```python
from build123d import *

# Parameters (mm, degrees)
SKETCH1_R           = 51.5
BOSS_EXTRUDE1_DEPTH = 2
SKETCH2_R           = 17.25
CUT_EXTRUDE1_DEPTH  = 2
BOSS_EXTRUDE3_START = 6
BOSS_EXTRUDE3_DEPTH = 6
CIRPATTERN2_COUNT   = 6
BOSS_EXTRUDE4_START = 6
SKETCH5_R           = 19.5
SKETCH5_R_2         = 17.25
BOSS_EXTRUDE4_DEPTH = 6
CHAMFER1_SIZE       = 1
CHAMFER1_SIZE2      = 3
BOSS_EXTRUDE5_START = 2
SKETCH6_R           = 51.5
BOSS_EXTRUDE5_DEPTH = 2
SKETCH7_R           = 19.5
BOSS_EXTRUDE6_DEPTH = 5
SKETCH8_R           = 9.5
BOSS_EXTRUDE7_DEPTH = 28
CUT_EXTRUDE2_DEPTH  = 79.028840822
SKETCH10_R          = 7.5
CUT_EXTRUDE3_DEPTH  = 2
SKETCH11_R          = 15.5
SKETCH11_R_2        = 12.5
CUT_EXTRUDE4_DEPTH  = 3
SKETCH12_R          = 57.826662367
SKETCH12_R_2        = 50.5
CUT_EXTRUDE5_DEPTH  = 50


with BuildPart() as part:
    # Sketch1 → Boss-Extrude1 (new body)
    with BuildSketch(Plane.XY):
        Circle(SKETCH1_R)
    extrude(amount=BOSS_EXTRUDE1_DEPTH)

    # Sketch2 → Cut-Extrude1 (cut)
    with BuildSketch(Plane.XY.offset(2)):
        Circle(SKETCH2_R)
    extrude(amount=-CUT_EXTRUDE1_DEPTH, mode=Mode.SUBTRACT)

    # Sketch4 → Boss-Extrude3 (add)
    with BuildSketch(Plane(origin=(0, 0, 0), x_dir=(-1, 0, 0), z_dir=(0, 0, -1)).offset(BOSS_EXTRUDE3_START)):
        with BuildLine():
            Line((15.659504395, 12.715698759), (12.020980416, 14.553474713))
            ThreePointArc((12.020980416, 14.553474713), (-0.569243838, 34.9508437), (-21.374545455, 46.854869615))
            ThreePointArc((-21.374545455, 46.854869615), (-19.207405538, 47.784156082), (-17, 48.613269793))
            ThreePointArc((-17, 48.613269793), (3.810982012, 34.741493963), (15.659504395, 12.715698759))
        make_face()
    boss_extrude3 = extrude(amount=-BOSS_EXTRUDE3_DEPTH)

    # CirPattern2: Boss-Extrude3 ×6 about axis
    cirpattern2_axis = Axis((0, 0, 0), (0, 0, 1))
    for i in range(1, CIRPATTERN2_COUNT):
        add(boss_extrude3.rotate(cirpattern2_axis, i * 360 / CIRPATTERN2_COUNT))

    # Sketch5 → Boss-Extrude4 (add)
    with BuildSketch(Plane.XY.offset(2).offset(BOSS_EXTRUDE4_START)):
        Circle(SKETCH5_R)
        Circle(SKETCH5_R_2, mode=Mode.SUBTRACT)
    extrude(amount=-BOSS_EXTRUDE4_DEPTH)

    # Chamfer1
    chamfer1_edges = [part.edges().sort_by_distance(p)[0] for p in [
        (-17.25, 0, 8),
    ]]
    chamfer1_side = [part.faces().sort_by_distance(p)[0] for p in [
        (-18.948456711, 0, 8),
    ]]
    chamfer(chamfer1_edges, length=CHAMFER1_SIZE, length2=CHAMFER1_SIZE2, reference=chamfer1_side[0])

    # Sketch6 → Boss-Extrude5 (add)
    with BuildSketch(Plane(origin=(0, 0, -6), x_dir=(-1, 0, 0), z_dir=(0, 0, -1)).offset(BOSS_EXTRUDE5_START)):
        Circle(SKETCH6_R)
    extrude(amount=-BOSS_EXTRUDE5_DEPTH)

    # Sketch7 → Boss-Extrude6 (add)
    with BuildSketch(Plane(origin=(0, 0, -8), x_dir=(-1, 0, 0), z_dir=(0, 0, -1))):
        with Locations(Location((0, 0, 0), (0, 0, 180))):
            Circle(SKETCH7_R)
    extrude(amount=BOSS_EXTRUDE6_DEPTH)

    # Sketch8 → Boss-Extrude7 (add)
    with BuildSketch(Plane(origin=(0, 0, -13), x_dir=(-1, 0, 0), z_dir=(0, 0, -1))):
        Circle(SKETCH8_R)
    extrude(amount=-BOSS_EXTRUDE7_DEPTH)

    # Sketch9 → Cut-Extrude2 (cut, through all)
    with BuildSketch(Plane.XY.offset(15)):
        with BuildLine():
            Line((6, 0), (6, 3.605551275))
            ThreePointArc((6, 3.605551275), (0, 7), (-6, 3.605551275))
            Line((-6, 3.605551275), (-6, 0))
            Line((-6, 0), (-6, -3.605551275))
            ThreePointArc((-6, -3.605551275), (0, -7), (6, -3.605551275))
            Line((6, -3.605551275), (6, 0))
        make_face()
    extrude(amount=-CUT_EXTRUDE2_DEPTH, mode=Mode.SUBTRACT)

    # Sketch10 → Cut-Extrude3 (cut)
    with BuildSketch(Plane(origin=(0, 0, -13), x_dir=(-1, 0, 0), z_dir=(0, 0, -1))):
        Circle(SKETCH10_R)
    extrude(amount=-CUT_EXTRUDE3_DEPTH, mode=Mode.SUBTRACT)

    # Sketch11 → Cut-Extrude4 (cut)
    with BuildSketch(Plane(origin=(0, 0, -13), x_dir=(-1, 0, 0), z_dir=(0, 0, -1))):
        Circle(SKETCH11_R)
        Circle(SKETCH11_R_2, mode=Mode.SUBTRACT)
    extrude(amount=-CUT_EXTRUDE4_DEPTH, mode=Mode.SUBTRACT)

    # Sketch12 → Cut-Extrude5 (cut)
    with BuildSketch(Plane.XY.offset(-6)):
        Circle(SKETCH12_R)
        with Locations(Location((0, 0, 0), (0, 0, 6.803897331))):
            Circle(SKETCH12_R_2, mode=Mode.SUBTRACT)
    extrude(amount=-CUT_EXTRUDE5_DEPTH, mode=Mode.SUBTRACT)


solid = part.part
```
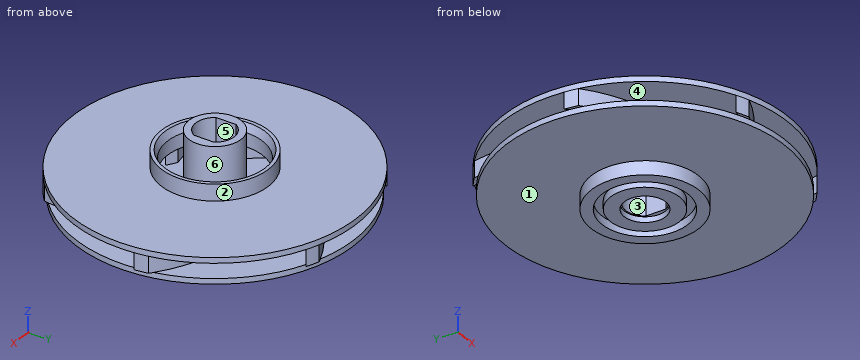
Geometry: final body of the model. Coordinates: model frame, mm. Face numbers are marked on the shaded views. A direction names the side the tool comes from. Coordinates: 2 decimals unless noted, no trailing zeros. Order: outer loops, then holes, each group sorted by start corner. A loop starts at its lowest first (then second) coordinate and runs counter-clockwise, first axis right, second up. Notation, with made-up numbers: (39, 77.5) -> (92, 77.5) arc R22 ccw to (92, 108.5) -> close; hole circle Ø8 at (41.5, 64). An arc over 180 degrees is marked (long way). Use CSV: the item, a comma, the result in double quotes.
1) Section B-B on z = 11. Output: boundary loops of the cut face in (x, y).
Findings:
outline,"circle Ø19 at (0, 0); hole (-6, -3.61) arc R7 ccw to (6, -3.61) -> (6, 3.61) arc R7 ccw to (-6, 3.61) -> close"
2) Section D-D on x = -38. Output: boundary loops of the cut face in (y, z).
Findings:
outline,"(-34.76, 0) -> (-17.47, 0) -> (-17.47, -6) -> (-33.26, -6) -> (-33.26, -8) -> (33.26, -8) -> (33.26, -6) -> (-14.18, -6) -> (-14.18, 0) -> (34.76, 0) -> (34.76, 2) -> (-34.76, 2) -> close"
3) Pin query (flat end, axial travel): pin 1 Ø2 at (x, y) = (32, -40.5) entering from -Z; pin 2 Ø5 at (x, y) = (24, -11.5) entering from -Z; pin 3 Ø4 at (x, z) = (-4.5, 11) entering from +Y. Return the tip coordinate at first contact, or that it passes through.
Findings:
pin 1,"stops at z = -6"
pin 2,"stops at z = -8"
pin 3,"stops at y = 9.17"
4) Access query for the marked faces 4, 5 and 6. Directions: +Z, -Z, +X, -X, +Y, -Y. A direction counts if a zero-diameter tool reaches every point of the face in a straight line with its end or side. Return the directions, or none.
Findings:
face 4,"none"
face 5,"+Z, -Z"
face 6,"+Z"
5) Mould query, pull axis X, two halves, no side actions, for the marked faces 1, 2 and 3. Classes: +X half, -X half, draft (parallel to the pull), parting line (faces both ways), or undercut.
Findings:
face 1,"draft"
face 2,"parting line"
face 3,"undercut"
6) Section C-C on x = 41. Output: boundary loops of the cut face in (y, z), then the cut area to 3 significant figures.
Findings:
outline,"(-31.16, 0) -> (12.63, 0) -> (12.63, -6) -> (-29.48, -6) -> (-29.48, -8) -> (29.48, -8) -> (29.48, -6) -> (16.04, -6) -> (16.04, 0) -> (31.16, 0) -> (31.16, 2) -> (-31.16, 2) -> close"
area,"263 mm^2"
7) Section A-A on y = 31.5. Output: boundary loops of the cut face in (x, z).
Findings:
outline,"(-40.74, 0) -> (-34.41, 0) -> (-34.41, -6) -> (-39.47, -6) -> (-39.47, -8) -> (39.47, -8) -> (39.47, -6) -> (-2.67, -6) -> (-2.67, 0) -> (40.74, 0) -> (40.74, 2) -> (-40.74, 2) -> close; hole (-31.41, -6) -> (-6.53, -6) -> (-6.53, 0) -> (-31.41, 0) -> close"
8) Line query: line 1 (Y direction, x = 0, z = -11.7); line 2 (Z direction, x = 20, y = -8); line 3 (X direction, y = 5, z = 5.5). Output: solid intervals per line, ascending.
Findings:
line 1,"y = -19.5 to -15.5, -12.5 to -7.5, 7.5 to 12.5, 15.5 to 19.5"
line 2,"z = -8 to -6, 0 to 2"
line 3,"x = -18.85 to -16.68, -8.08 to -4.9, 4.9 to 8.08, 16.68 to 18.85"
